Could you check a few things on this model? Use its own coordinates, in mm. A direction names the side the tool comes from. Round coordinates to 2 decimals unless told otherwise and drop trailing zeros. Write each loop counter-clockwise with the first axis right and the second up, starting at its lowest first coordinate (ties: lowest second). Pieces come first, ordered by that corner, then holes. Notation, with made-up numbers: M 2.25,47.25 L 44.25,47.25 A29 ccw 44.25,71.25 Z; hole C 26,38 d9. An arc over 180 degrees is marked long. One line per item, written item: value. Start each with the question number.
(1) I want a section at C-C on x = 9. Please give me the cut outline in (y, z).
(2) If I drill on L1, parallel to X at y = 7.5, z = 20; L2, parallel to Z at x = -29, y = 2.75, over which ranges is the centre line in solid material (lowest first)?
(3) I want a section at A-A on z = -21. Please give me the cut outline in (x, y), and give its area (3 significant figures).
(4) Thinking about a two-plate mould opening in X: for faces 1 (the face through (-15, 5, -22)), 2 (the face through (-35, 5, -2)), 3 (the face through (20, 5, -25)), which applies, released by +X, released by -X, zero draft, split by the parting line, or undercut?
(5) I want a section at B-B on y = 5.75. Please give me the cut outline in (x, z).
(6) Which directions (+Z, -Z, +X, -X, +Y, -Y) give clear straight access to the entire face, cutting with the end or side of a thin tool? Please do faces 4 (the face through (-5, 5, -22)), 5 (the face through (10, 5, 15)), 6 (the face through (25, 5, -22)).
(7) I'm going to push flat-ended pins straight in: pin 1 Ø8 at (x, z) = (-11.5, 18) entering from -Y; pin 2 Ø3 at (y, z) = (5.5, 21.5) entering from -X; pin 3 Ø5 at (x, y) = (11.5, 3.5) entering from +Z; pin 4 Ø5 at (y, z) = (5, 19) entering from +X. Where does each tip first touch, or does it pass through?
```python
from build123d import *

# Parameters (mm, degrees)
SKETCH1_W           = 70
SKETCH1_H           = 50
BOSS_EXTRUDE1_DEPTH = 10
SKETCH2_W           = 10
SKETCH2_H           = 5
SKETCH2_H_2         = 10
CUT_EXTRUDE1_DEPTH  = 45.158804332
LPATTERN1_COUNT     = 4
LPATTERN1_PITCH     = 20


with BuildPart() as part:
    # Sketch1 → Boss-Extrude1 (new body)
    with BuildSketch(Plane(origin=(0, 0, 0), x_dir=(1, 0, 0), z_dir=(0, 1, 0))):
        Rectangle(SKETCH1_W, SKETCH1_H)
    extrude(amount=BOSS_EXTRUDE1_DEPTH)

    # Sketch2 → Cut-Extrude1 (cut, through all)
    with BuildSketch(Plane(origin=(0, 10, 0), x_dir=(1, 0, 0), z_dir=(0, 1, 0))):
        with Locations((-30, 22.5)):
            Rectangle(SKETCH2_W, SKETCH2_H)
        with Locations((-30, -20)):
            Rectangle(SKETCH2_W, SKETCH2_H_2)
    cut_extrude1 = extrude(amount=-CUT_EXTRUDE1_DEPTH, mode=Mode.SUBTRACT)

    # LPattern1: Cut-Extrude1 ×4
    with Locations(*[(i * LPATTERN1_PITCH, 0, 0) for i in range(1, LPATTERN1_COUNT)]):
        add(cut_extrude1, mode=Mode.SUBTRACT)


solid = part.part
```
Found:
1. outline: M 0,-20 L 10,-20 L 10,15 L 0,15 Z
2. L1: x = -25 to -15, -5 to 5, 15 to 25
2. L2: z = -20 to 15
3. outline: M -25,0 L -15,0 L -15,10 L -25,10 Z; M -5,0 L 5,0 L 5,10 L -5,10 Z; M 15,0 L 25,0 L 25,10 L 15,10 Z
3. area: 300 mm²
4. face 1: undercut
4. face 2: released by -X
4. face 3: zero draft
5. outline: M -35,-20 L -25,-20 L -25,-25 L -15,-25 L -15,-20 L -5,-20 L -5,-25 L 5,-25 L 5,-20 L 15,-20 L 15,-25 L 25,-25 L 25,-20 L 35,-20 L 35,15 L 25,15 L 25,25 L 15,25 L 15,15 L 5,15 L 5,25 L -5,25 L -5,15 L -15,15 L -15,25 L -25,25 L -25,15 L -35,15 Z
6. face 4: -Z, +Y, -Y
6. face 5: +Z, +Y, -Y
6. face 6: -Z, +X, +Y, -Y
7. pin 1: stops at y = 0
7. pin 2: stops at x = -25
7. pin 3: stops at z = 15
7. pin 4: stops at x = 25
